from build123d import *

# Parameters (mm, degrees)
SKETCH1_R           = 5
SKETCH1_R_2         = 2
BOSS_EXTRUDE1_DEPTH = 2
SKETCH2_R           = 2
SKETCH2_R_2         = 5
BOSS_EXTRUDE2_DEPTH = 2
BOSS_EXTRUDE3_DEPTH = 46
SKETCH7_R           = 3
SKETCH7_R_2         = 2.5
BOSS_EXTRUDE4_DEPTH = 46
BOSS_EXTRUDE5_DEPTH = 46
SKETCH10_R          = 5
SKETCH10_R_2        = 2.5
BOSS_EXTRUDE6_DEPTH = 5


with BuildPart() as part:
    # Sketch1 → Boss-Extrude1 (new body)
    with BuildSketch(Plane.XY):
        with BuildLine():
            Line((-25, 0), (25, 0))
            Line((25, 0), (14.104686356, 30.104686356))
            ThreePointArc((14.104686356, 30.104686356), (0, 40), (-14.104686356, 30.104686356))
            Line((-14.104686356, 30.104686356), (-25, 0))
        make_face()
        with Locations((0, 20)):
            Circle(SKETCH1_R, mode=Mode.SUBTRACT)
        with Locations((-10, 8)):
            Circle(SKETCH1_R_2, mode=Mode.SUBTRACT)
        with Locations((10, 8)):
            Circle(SKETCH1_R_2, mode=Mode.SUBTRACT)
        with Locations((0, 33)):
            Circle(SKETCH1_R_2, mode=Mode.SUBTRACT)
    extrude(amount=BOSS_EXTRUDE1_DEPTH)



with BuildPart() as body_2:
    # Sketch2 → Boss-Extrude2 (new body)
    with BuildSketch(Plane(origin=(0, 0, 50), x_dir=(-1, 0, 0), z_dir=(0, 0, -1))):
        with BuildLine():
            Line((-25, 0), (25, 0))
            Line((25, 0), (14.104686356, 30.104686356))
            ThreePointArc((14.104686356, 30.104686356), (0, 40), (-14.104686356, 30.104686356))
            Line((-14.104686356, 30.104686356), (-25, 0))
        make_face()
        with Locations(Location((-10, 8, 0), (0, 0, 180))):
            Circle(SKETCH2_R, mode=Mode.SUBTRACT)
        with Locations(Location((10, 8, 0), (0, 0, 180))):
            Circle(SKETCH2_R, mode=Mode.SUBTRACT)
        with Locations(Location((0, 33, 0), (0, 0, 180))):
            Circle(SKETCH2_R, mode=Mode.SUBTRACT)
        with Locations(Location((0, 20, 0), (0, 0, 180))):
            Circle(SKETCH2_R_2, mode=Mode.SUBTRACT)
    extrude(amount=BOSS_EXTRUDE2_DEPTH)


with BuildPart() as part_1:
    add(part.part)

    add(body_2.part)  # Boss-Extrude3 merges body 2
    # Sketch4 → Boss-Extrude3 (add)
    with BuildSketch(Plane(origin=(0, 0, 48), x_dir=(-1, 0, 0), z_dir=(0, 0, -1))):
        Polygon((-25, 0), (25, 0), (23.552343178, 4), (-23.552343178, 4), align=None)
    extrude(amount=BOSS_EXTRUDE3_DEPTH)

    # Sketch7 → Boss-Extrude4 (add)
    # profile 1 of 3: a face of its own
    with BuildSketch(Plane(origin=(0, 0, 48), x_dir=(-1, 0, 0), z_dir=(0, 0, -1))):
        with Locations(Location((10, 8, 0), (0, 0, 180))):
            Circle(SKETCH7_R)
        with Locations(Location((10, 8, 0), (0, 0, 180))):
            Circle(SKETCH7_R_2, mode=Mode.SUBTRACT)
    # profile 2 of 3: a face of its own
    with BuildSketch(Plane(origin=(0, 0, 48), x_dir=(-1, 0, 0), z_dir=(0, 0, -1))):
        with Locations(Location((0, 33, 0), (0, 0, 180))):
            Circle(SKETCH7_R)
        with Locations(Location((0, 33, 0), (0, 0, 180))):
            Circle(SKETCH7_R_2, mode=Mode.SUBTRACT)
    # profile 3 of 3: a face of its own
    with BuildSketch(Plane(origin=(0, 0, 48), x_dir=(-1, 0, 0), z_dir=(0, 0, -1))):
        with Locations(Location((-10, 8, 0), (0, 0, 180))):
            Circle(SKETCH7_R)
        with Locations(Location((-10, 8, 0), (0, 0, 180))):
            Circle(SKETCH7_R_2, mode=Mode.SUBTRACT)
    extrude(amount=BOSS_EXTRUDE4_DEPTH)

    # Sketch5 → Boss-Extrude5 (add)
    with BuildSketch(Plane(origin=(0, 0, 48), x_dir=(-1, 0, 0), z_dir=(0, 0, -1))):
        Polygon((19.298437881, 4), (9.850781059, 30.104686356), (14.104686356, 30.104686356), (23.552343178, 4), align=None)
        Polygon((-23.552343178, 4), (-19.298437881, 4), (-9.850781059, 30.104686356), (-14.104686356, 30.104686356), align=None)
    extrude(amount=BOSS_EXTRUDE5_DEPTH)

    # Sketch10 → Boss-Extrude6 (add)
    # profile 1 of 4: a face of its own
    with BuildSketch(Plane.XZ):
        with Locations(Location((-12.5, 12.5, 0), (0, 0, 90))):
            Circle(SKETCH10_R)
        with Locations(Location((-12.5, 12.5, 0), (0, 0, 270))):
            Circle(SKETCH10_R_2, mode=Mode.SUBTRACT)
    # profile 2 of 4: a face of its own
    with BuildSketch(Plane.XZ):
        with Locations(Location((-12.5, 37.5, 0), (0, 0, 90))):
            Circle(SKETCH10_R)
        with Locations(Location((-12.5, 37.5, 0), (0, 0, 90))):
            Circle(SKETCH10_R_2, mode=Mode.SUBTRACT)
    # profile 3 of 4: a face of its own
    with BuildSketch(Plane.XZ):
        with Locations(Location((12.5, 37.5, 0), (0, 0, 90))):
            Circle(SKETCH10_R)
        with Locations(Location((12.5, 37.5, 0), (0, 0, 270))):
            Circle(SKETCH10_R_2, mode=Mode.SUBTRACT)
    # profile 4 of 4: a face of its own
    with BuildSketch(Plane.XZ):
        with Locations(Location((12.5, 12.5, 0), (0, 0, 90))):
            Circle(SKETCH10_R)
        with Locations(Location((12.5, 12.5, 0), (0, 0, 90))):
            Circle(SKETCH10_R_2, mode=Mode.SUBTRACT)
    extrude(amount=BOSS_EXTRUDE6_DEPTH)


solid = part_1.part
Source: CAD feature listing. Evaluate the final solid. Frame: model axes, mm. A direction names the side the tool comes from. Round coordinates to 2 decimals unless told otherwise and drop trailing zeros. Loops run counter-clockwise (first coordinate to the right, second up) from the corner with the lowest first, then second, coordinate; pieces in that order, holes last. Notation, with made-up numbers: M 77,-36.75 L 91,-36.75 A8 ccw 91,-27.75 Z; hole C 3.25,37 d10. An arc over 180 degrees is marked long. Return JSON: item names as keys, results as strings. Group by question number.
1. Section query B-B on z = 31. Output: boundary loops of the cut face in (x, y).
2. Section query D-D on y = 33. Output: boundary loops of the cut face in (x, z).
3. Pin query (flat end, axial travel): pin 1 (6 mm diameter, centred on x = -10, z = 33.5, fed in from +Y); pin 2 (1.5 mm diameter, centred on y = 23, z = 28, fed in from +X); pin 3 (1.5 mm diameter, centred on y = 5, z = 40, fed in from +X). Return the tip coordinate at first contact, or that it passes through.
4. Mould query, pull axis Z, two halves, no side actions, for faces 6 (the face through (14, -5, 10)), 7 (the face through (9.46, 10.44, 25.32)), 8 (the face through (-5, 22, 2)), 9 (the face through (5, 16, 0)). Classes: released by +Z, released by -Z, zero draft, split by the parting line, or undercut.
5. Section query A-A on y = -1.5. Output: boundary loops of the cut face in (x, z), and give its area (3 significant figures).
6. Reachability of faces 1 (the face through (12.86, 7.1, 25.32)), 2 (the face through (13, 0, 13)), 3 (the face through (-11.474, 6.648, 49.014)), 4 (the face through (-5, 16, 50)), 5 (the face through (12, 30.105, 25)) from +Z, -Z, +X, -X, +Y, -Y: full face, straight path, thin tool, end or side. Return the list, or none.
7. Section query C-C on x = 0. State how many separate pieces and enclosed holes the cut face has, and give its area (3 significant figures).
8. Material intervals for line 1 along Y through (x, z) = (0, 1); line 2 along Z through (x, y) = (9, 13); line 3 along X through (y, z) = (-0.5, 14), sorted ascending. Write a range as from..to.
Checks:
{
 "1": {"outline": "M -25,0 L 25,0 L 14.1,30.1 L 9.85,30.1 L 19.3,4 L -19.3,4 L -9.85,30.1 L -14.1,30.1 Z; C -10,8 d6; C 0,33 d6; C 10,8 d6; hole C -10,8 d5; hole C 0,33 d5; hole C 10,8 d5"},
 "2": {"outline": "M -12.69,0 L -2,0 L -2,2 L -2.5,2 L -2.5,48 L -2,48 L -2,50 L -12.69,50 L -12.69,48 L -3,48 L -3,2 L -12.69,2 Z; M 2,0 L 12.69,0 L 12.69,2 L 3,2 L 3,48 L 12.69,48 L 12.69,50 L 2,50 L 2,48 L 2.5,48 L 2.5,2 L 2,2 Z"},
 "3": {"pin 1": "stops at y = 30.1", "pin 2": "stops at x = 16.95", "pin 3": "stops at x = 23.46"},
 "4": {"face 6": "zero draft", "face 7": "undercut", "face 8": "undercut", "face 9": "released by -Z"},
 "5": {"outline": "C -12.5,12.5 d10; C -12.5,37.5 d10; C 12.5,12.5 d10; C 12.5,37.5 d10; hole C -12.5,12.5 d5; hole C -12.5,37.5 d5; hole C 12.5,12.5 d5; hole C 12.5,37.5 d5", "area": "236 mm²"},
 "6": {"face 1": "none", "face 2": "-Y", "face 3": "+Z, -Z", "face 4": "+Z, +X, -X, +Y, -Y", "face 5": "+X, +Y"},
 "7": {"separate pieces": "3", "enclosed holes": "0", "area": "334 mm²"},
 "8": {"line 1": "y = 0..15, 25..31, 35..40", "line 2": "z = 0..2, 48..50", "line 3": "x = -17.27..-14.5, -10.5..-7.73, 7.73..10.5, 14.5..17.27"}
}
